from build123d import *

# Parameters (mm, degrees)
SKETCH_1_R          = 4
EXTRUDE_1_DEPTH     = 8
SKETCH_2_R          = 3.5
EXTRUDE_2_DEPTH     = 40
CHAMFER_1_SIZE      = 1.5
CHAMFER_1_SIZE_2    = 2.598076211
SKETCH_3_R          = 2
CUT_EXTRUDE_1_DEPTH = 101
CHAMFER_2_SIZE      = 1
CHAMFER_2_SIZE2     = 2.747477419


with BuildPart() as part:
    # 草图1 → 凸台-拉伸1 (new body)
    with BuildSketch(Plane(origin=(0, 0, 0), x_dir=(1, 0, 0), z_dir=(0, 1, 0))):
        with Locations(Location((0, 0, 0), (0, 0, 270))):
            Circle(SKETCH_1_R)
    extrude(amount=EXTRUDE_1_DEPTH)

    # 草图2 → 凸台-拉伸2 (add)
    with BuildSketch(Plane.XZ):
        with Locations(Location((0, 0, 0), (0, 0, 270))):
            Circle(SKETCH_2_R)
    extrude(amount=EXTRUDE_2_DEPTH)

    # 倒角1
    # the kernel refuses this chamfer: 2.598076211, 1.5 mm, written as the material it adds along each edge
    with BuildSketch(Plane(origin=(0, 0, 0), x_dir=(0, 0, -1), z_dir=(-1, 0, 0))) as chamfer_1_piece_1_section:
        Polygon((3.5 + CHAMFER_1_SIZE, 0), (3.5, CHAMFER_1_SIZE_2), (3.5, 0), align=None)
    chamfer_1_piece_1 = revolve(axis=Axis((0, 0, 0), (0, -1, 0)), mode=Mode.PRIVATE)
    chamfer_1_piece_1 = chamfer_1_piece_1 & Plane(origin=(0, -2.194625368, 0), x_dir=(0, 0, 1), z_dir=(0, -1, 0)) * Cylinder(4, 20, mode=Mode.PRIVATE)
    add(chamfer_1_piece_1)

    # 草图3 → 切除-拉伸1 (cut)
    with BuildSketch(Plane.XZ.offset(40)):
        with Locations(Location((0, 0, 0), (0, 0, 270))):
            Circle(SKETCH_3_R)
    extrude(amount=-CUT_EXTRUDE_1_DEPTH, mode=Mode.SUBTRACT)

    # 倒角2
    chamfer_2_edges = [part.edges().sort_by_distance(p)[0] for p in [
        (0, 8, 2),
    ]]
    chamfer_2_side = [part.faces().sort_by_distance(p)[0] for p in [
        (0, 8, -3.886862915),
    ]]
    chamfer(chamfer_2_edges, length=CHAMFER_2_SIZE, length2=CHAMFER_2_SIZE2, reference=chamfer_2_side[0])


solid = part.part
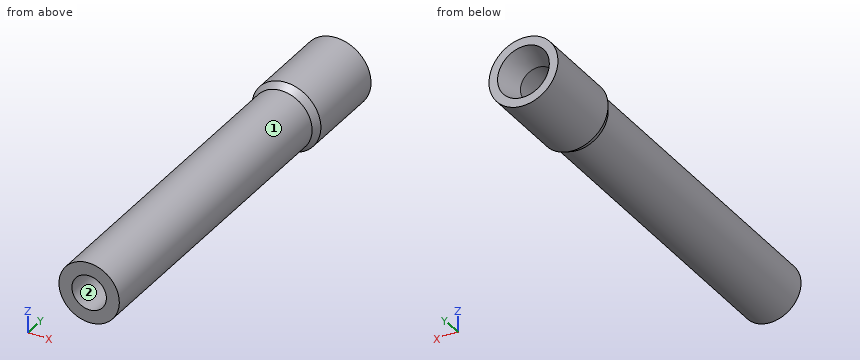
Design review of the part built by this model. Coordinates are the model's own, in mm. Face numbers are marked on the shaded views. Give positions to 0.01 mm unless a question says otherwise; leave off trailing zeros. Loops run counter-clockwise (first coordinate to the right, second up) from the corner with the lowest first, then second, coordinate; pieces in that order, holes last. Notation, with made-up numbers: (67.25, -39.75) - (122.25, -39.75) arc R25 ccw to (122.25, -27.75) - close; hole circle Ø2 at (70.25, 41.25). An arc over 180 degrees is marked (long way). Write item = value, one per line.
1) To check wall thickness, follow line 1 (X direction, y = -12, z = 0); line 2 (Z direction, x = 1.5, y = -18.5); line 3 (X direction, y = -33.5, z = -0.5). State the ranges of each line that lie inside material, in increasing order.
Result sheet:
line_1 = -3.5 to -2, 2 to 3.5
line_2 = -3.16 to -1.32, 1.32 to 3.16
line_3 = -3.46 to -1.94, 1.94 to 3.46
2) Take a section at B-B on x = 0. State the section outline as (y, z) points.
Result sheet:
outline = (-40, -3.5) - (-2.6, -3.5) - (-1.73, -4) - (8, -4) - (8, -3) - (5.25, -2) - (-40, -2) - close; (-40, 2) - (5.25, 2) - (8, 3) - (8, 4) - (-1.73, 4) - (-2.6, 3.5) - (-40, 3.5) - close
3) Take a section at A-A on z = 0. State the section outline as (x, y) points, and give its area (3 significant figures).
Result sheet:
outline = (-4, -1.73) - (-3.5, -2.6) - (-3.5, -40) - (-2, -40) - (-2, 5.25) - (-3, 8) - (-4, 8) - close; (2, -40) - (3.5, -40) - (3.5, -2.6) - (4, -1.73) - (4, 8) - (3, 8) - (2, 5.25) - close
area = 151 mm2
4) Draft analysis for pull direction X (two halves, no side actions). For the marked faces 1 and 2, state which applies: +X half, -X half, draft (parallel to the pull), parting line (faces both ways), or undercut.
Result sheet:
face_1 = parting line
face_2 = undercut
5) Take a section at C-C on y = 4. State the section outline as (x, z) points.
Result sheet:
outline = circle Ø8 at (0, 0); hole circle Ø4 at (0, 0)
6) Clearance check with flat-ended pins moving along their axes: pin 1 Ø3 at (y, z) = (-26.5, 0.5) entering from +X; pin 2 Ø4 at (x, y) = (2, -1.5) entering from -Z. State where each tip first meets the part, or that it passes through.
Result sheet:
pin_1 = 3.5
pin_2 = -4
7) Take a section at D-D on y = -6. State the section outline as (x, z) points.
Result sheet:
outline = circle Ø7 at (0, 0); hole circle Ø4 at (0, 0)
